Input: part model. Units: mm. Frame: model coordinates. Face numbers are marked on the shaded views. A direction names the side the tool comes from. Coordinates: 2 decimals unless noted, no trailing zeros. Write each loop counter-clockwise with the first axis right and the second up, starting at its lowest first coordinate (ties: lowest second). Pieces come first, ordered by that corner, then holes. Notation, with made-up numbers: M 53,8 L 105,8 A6 ccw 105,16 Z; hole C 59,69 d7. An arc over 180 degrees is marked long. Write each question's results on one line, items separated by ' | '. Start each with the question number.
1. First-contact query: pin 1 (6 mm diameter, centred on x = 4.5, z = 1.5, fed in from +Y); pin 2 (3 mm diameter, centred on x = 7.5, y = 0, fed in from +Z); pin 3 (2.5 mm diameter, centred on y = 0, z = 1, fed in from -X). Flat tips, straight axial feed; report the tip coordinate or a pass-through.
2. Section query A-A, the plane x = -0.5. Output: boundary loops of the cut face in (y, z), and give its area (3 significant figures).
3. Set-up query: the marked faces 1 and 2. Return all of +Z, -Z, +X, -X, +Y, -Y with unobstructed straight access to the full face (end or side cutting, diameter ignored); none if empty.
4. Section query B-B, the plane x = 5. Output: boundary loops of the cut face in (y, z).
5. Pull-direction query (Y, two-part tool) for the marked faces 3, 4, 5 and 6; classes: +Y half, -Y half, draft (parallel to the pull), parting line (faces both ways), or undercut.
6. Ray query, probe 1 along X at (y, z) = (-2.5, 2); probe 2 along Z at (x, y) = (-3.75, -2.5); probe 3 along Y at (x, z) = (-1.5, -4). Return the intervals inside material, ascending.
```python
from build123d import *

# Parameters (mm, degrees)
CUT_EXTRUDE1_DEPTH = 3
CHAMFER1_SIZE      = 0.5


with BuildPart() as part:
    # Sketch1 → Revolve1 (revolve)
    with BuildSketch(Plane.XY, mode=Mode.PRIVATE) as revolve1_sk:
        Polygon((-6, 0), (-6, 5), (0, 5), (0, 3), (12, 3), (12, 0), align=None)
    revolve(revolve1_sk.sketch.rotate(Axis((12, 0, 0), (-1, 0, 0)), 180), axis=Axis((12, 0, 0), (-1, 0, 0)))

    # Sketch2 → Cut-Revolve1 (revolve, cut)
    with BuildSketch(Plane.XY, mode=Mode.PRIVATE) as cut_revolve1_sk:
        Polygon((-6, 0), (-6, 2.495), (-3, 2.495), (-2.331466765, 0), align=None)
    revolve(cut_revolve1_sk.sketch.rotate(Axis((-2.331466765, 0, 0), (-1, 0, 0)), 270), axis=Axis((-2.331466765, 0, 0), (-1, 0, 0)), mode=Mode.SUBTRACT)

    # Sketch3 → Cut-Extrude1 (cut)
    with BuildSketch(Plane.ZY.offset(6)):
        Polygon((0, 2.886751346), (-2.5, 1.443375673), (-2.5, -1.443375673), (0, -2.886751346), (2.5, -1.443375673), (2.5, 1.443375673), align=None)
    extrude(amount=-CUT_EXTRUDE1_DEPTH, mode=Mode.SUBTRACT)

    # Chamfer1
    chamfer1_edges = [part.edges().sort_by_distance(p)[0] for p in [
        (12, 3, 0),
        (-6, 5, 0),
    ]]
    chamfer(chamfer1_edges, length=CHAMFER1_SIZE)


solid = part.part
```
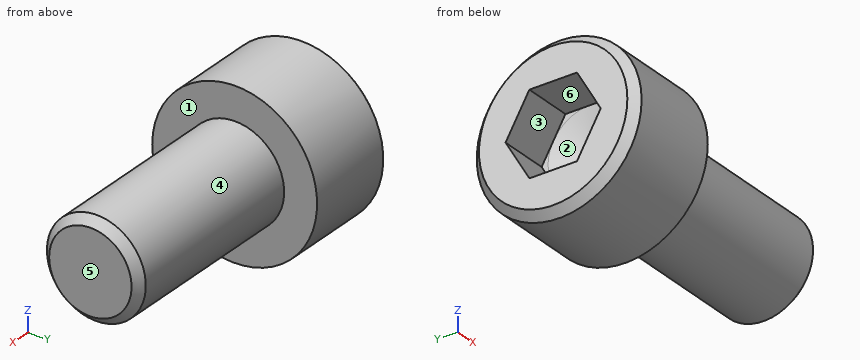
Answer:
1) pin 1: y = 3 | pin 2: z = 3 | pin 3: x = -2.93
2) outline: C 0,0 d10 | area: 78.5 mm^2
3) face 1: +X | face 2: -X
4) outline: C 0,0 d6
5) face 3: undercut | face 4: parting line | face 5: draft | face 6: undercut
6) probe 1: -6 to 0 | probe 2: -4.33 to -0.67, 0.67 to 4.33 | probe 3: -3 to 3
